Job drawing, mm, ordinate dimensions from the low corner. One solid piece. A direction names the side the tool comes from. Give positions to 0.01 mm unless a question says otherwise; leave off trailing zeros. Order: outer loops, then holes, each group sorted by start corner. A loop starts at its lowest first (then second) coordinate and runs counter-clockwise, first axis right, second up. Notation, with made-up numbers: (-6, -31) -> (39, -31) arc R22 cw to (39, 0) -> close; hole circle Ø11 at (8, 10.5). An arc over 180 degrees is marked (long way). Write item = value, one per line. Start each with the question number.
(1) Flat gauge pins, fed straight in: pin 1 (3 mm diameter, centred on x = 5, z = 5, fed in from -Y); pin 2 (1.5 mm diameter, centred on x = 5.5, z = 4, fed in from +Y); pin 3 (3 mm diameter, centred on x = 4.5, z = 6, fed in from +Y). Where does each tip first touch, or does it go through?
(2) Saw through at D-D, the plane x = 5.5. List the corners of the cut face in (y, z).
(3) Saw through at B-B, the plane y = 3. List the corners of the cut face in (x, z), then the cut area to 3 significant figures.
(4) Saw through at C-C, the plane z = 8.5. List the corners of the cut face in (x, y) (3 decimals).
(5) Probe line 1 along Z through (x, y) = (0.75, 4.75); line 2 along X through (y, z) = (2, 4.5); line 3 along Y through (x, z) = (3.5, 7.25). List the from-to ranges inside material, lowest first. Write a range as from..to.
(6) Which spindle directions (+Z, -Z, +X, -X, +Y, -Y) get a long thin tool onto all of the face, cutting with end or side? Do the marked faces 1 and 2. Say none if no direction does.
(7) Saw through at A-A, the plane x = 4. List the corners of the cut face in (y, z), then the cut area to 3 significant figures.
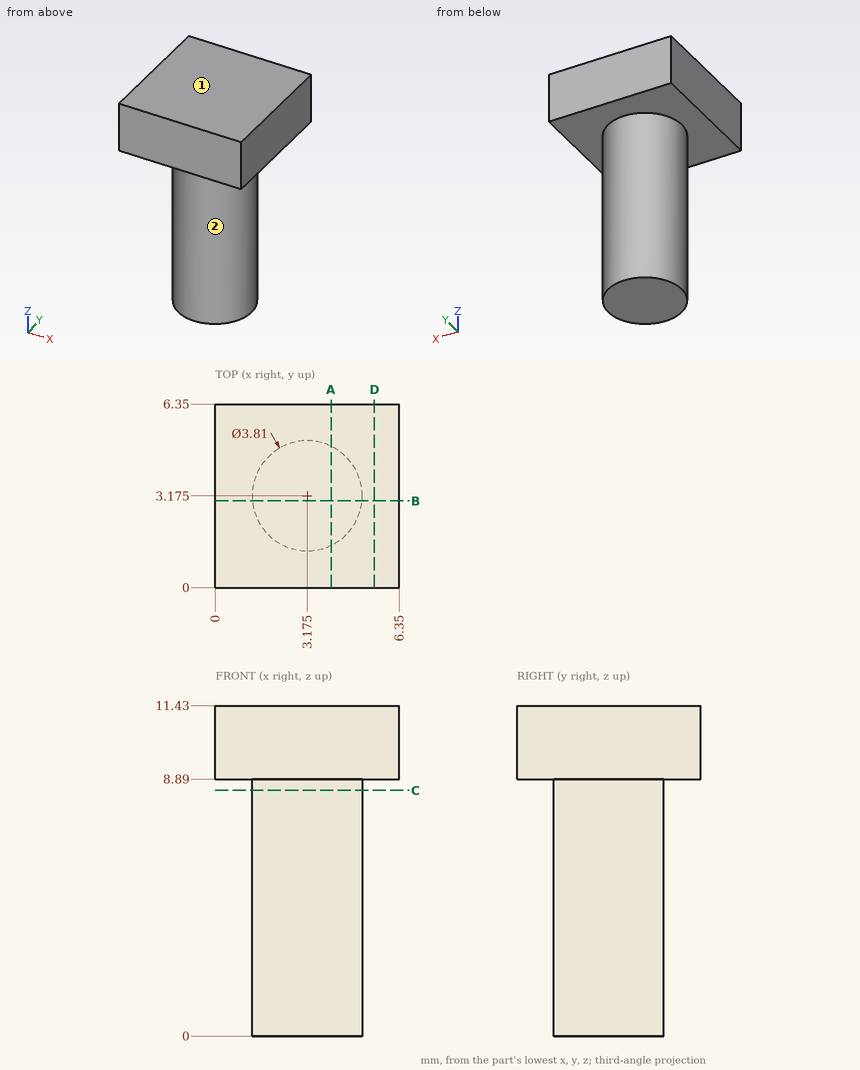
Results list:
q1.pin_1 = 1.3
q1.pin_2 = 4.25
q1.pin_3 = 5.08
q2.outline = (0, 8.89) -> (6.35, 8.89) -> (6.35, 11.43) -> (0, 11.43) -> close
q3.outline = (0, 8.89) -> (1.28, 8.89) -> (1.28, 0) -> (5.07, 0) -> (5.07, 8.89) -> (6.35, 8.89) -> (6.35, 11.43) -> (0, 11.43) -> close
q3.area = 49.9 mm^2
q4.outline = circle Ø3.81 at (3.175, 3.175)
q5.line_1 = 8.89..11.43
q5.line_2 = 1.68..4.67
q5.line_3 = 1.3..5.05
q6.face_1 = +Z, +X, -X, +Y, -Y
q6.face_2 = -Z
q7.outline = (0, 8.89) -> (1.46, 8.89) -> (1.46, 0) -> (4.89, 0) -> (4.89, 8.89) -> (6.35, 8.89) -> (6.35, 11.43) -> (0, 11.43) -> close
q7.area = 46.7 mm^2
